Here's how the part is built. I have some questions about the finished solid (model axes, mm). Face numbers are marked on the shaded views. A direction names the side the tool comes from. Coordinates: 2 decimals unless noted, no trailing zeros. Write each loop counter-clockwise with the first axis right and the second up, starting at its lowest first coordinate (ties: lowest second). Pieces come first, ordered by that corner, then holes.
(1) Thinking about a two-plate mould opening in X: for the marked faces 3, 4, 5 and 6, which applies, released by +X, released by -X, zero draft, split by the parting line, or undercut?
(2) For pin 1 Ø3 at (y, z) = (2.5, -25) entering from +X; pin 2 Ø5 at (x, y) = (0, 4.5) entering from +Z; pin 3 Ø1.9 at (x, z) = (-24.5, -20) entering from +Y, each with a flat end and sliding along its axis, tell me the tip position at first contact or that it passes through.
(3) Imagine slicing it at B-B, the plane x = -24.5. List the corners of the cut face in (y, z) for me.
(4) Imagine slicing it at C-C, the plane y = 4.75. List the corners of the cut face in (x, z) for me, plus the area to 3 significant figures.
(5) Imagine slicing it at D-D, the plane x = -45. List the corners of the cut face in (y, z) for me, plus the area to 3 significant figures.
(6) Imagine slicing it at A-A, the plane z = 2.5. List the corners of the cut face in (x, y) for me, plus the area to 3 significant figures.
(7) Please list where these lines run through material, in increasing order: probe 1 along Z at (x, y) = (-7.5, 1); probe 2 along X at (y, z) = (5, 10.5); probe 3 along X at (y, z) = (5.75, -15).
(8) Which directions (+Z, -Z, +X, -X, +Y, -Y) give clear straight access to the entire face, cutting with the end or side of a thin tool? Please do the marked faces 1 and 2.
```python
from build123d import *

# Parameters (mm, degrees)
SKETCH1_R           = 50
BOSS_EXTRUDE1_DEPTH = 10
CUT_EXTRUDE1_DEPTH  = 35
SKETCH5_W           = 35.6075
SKETCH5_H           = 50.6
CUT_EXTRUDE2_DEPTH  = 2.5
SKETCH7_R           = 4.5
CUT_EXTRUDE3_DEPTH  = 10
SKETCH7_3_R         = 4.5
CUT_EXTRUDE4_DEPTH  = 10
SKETCH7_4_R         = 4.5
CUT_EXTRUDE5_DEPTH  = 10


with BuildPart() as part:
    # Sketch1 → Boss-Extrude1 (new body)
    with BuildSketch(Plane(origin=(0, 0, 0), x_dir=(1, 0, 0), z_dir=(0, 1, 0))):
        with Locations(Location((-8.682864084, 10.831764098, 0), (0, 0, 270))):
            Circle(SKETCH1_R)
    extrude(amount=BOSS_EXTRUDE1_DEPTH)

    # Sketch2 → Cut-Extrude1 (cut)
    with BuildSketch(Plane(origin=(0, 10, 0), x_dir=(1, 0, 0), z_dir=(0, 1, 0))):
        with BuildLine():
            Line((-26.490364084, 15.731764356), (-26.492864056, -20.667823814))
            ThreePointArc((-26.492864056, -20.667823814), (-26.308368402, -21.704061868), (-25.777306707, -22.612798037))
            Line((-25.777306707, -22.612798037), (-22.287306707, -26.712798037))
            ThreePointArc((-22.287306707, -26.712798037), (-21.261099672, -27.491624086), (-20.002864084, -27.768235902))
            Line((-20.002864084, -27.768235902), (2.632135916, -27.768235902))
            ThreePointArc((2.632135916, -27.768235902), (3.890371505, -27.491624086), (4.91657854, -26.712798037))
            Line((4.91657854, -26.712798037), (8.40657854, -22.612798037))
            ThreePointArc((8.40657854, -22.612798037), (8.937569086, -21.704255238), (9.122135916, -20.668235902))
            Line((9.122135916, -20.668235902), (9.122135916, 15.721764098))
            ThreePointArc((9.122135916, 15.721764098), (8.938191307, 16.756090949), (8.40891456, 17.663578567))
            Line((8.40891456, 17.663578567), (4.91891456, 21.773578567))
            ThreePointArc((4.91891456, 21.773578567), (3.892008249, 22.554395492), (2.632135916, 22.831764098))
            Line((2.632135916, 22.831764098), (-19.997864084, 22.831764098))
            ThreePointArc((-19.997864084, 22.831764098), (-21.255584517, 22.555390231), (-22.28157091, 21.777190306))
            Line((-22.28157091, 21.777190306), (-25.774070917, 17.677396608))
            ThreePointArc((-25.774070917, 17.677396608), (-26.30563684, 16.768425583), (-26.490364084, 15.731764356))
        make_face()
    extrude(amount=-CUT_EXTRUDE1_DEPTH, mode=Mode.SUBTRACT)

    # Sketch5 → Cut-Extrude2 (cut)
    with BuildSketch(Plane(origin=(0, 10, 0), x_dir=(1, 0, 0), z_dir=(0, 1, 0))):
        with Locations((-8.686614084, -2.468235902)):
            Rectangle(SKETCH5_W, SKETCH5_H)
    extrude(amount=-CUT_EXTRUDE2_DEPTH, mode=Mode.SUBTRACT)

    # Sketch7 → Cut-Extrude3 (cut)
    with BuildSketch(Plane(origin=(0, 10, 0), x_dir=(1, 0, 0), z_dir=(0, 1, 0))):
        with Locations(Location((26.391164769, -9.418235902, 0), (0, 0, 270))):
            Circle(SKETCH7_R)
    extrude(amount=-CUT_EXTRUDE3_DEPTH, mode=Mode.SUBTRACT)

    # Sketch7_3 → Cut-Extrude4 (cut)
    with BuildSketch(Plane(origin=(0, 10, 0), x_dir=(1, 0, 0), z_dir=(0, 1, 0))):
        with Locations(Location((-43.756892937, -9.418235902, 0), (0, 0, 270))):
            Circle(SKETCH7_3_R)
    extrude(amount=-CUT_EXTRUDE4_DEPTH, mode=Mode.SUBTRACT)

    # Sketch7_4 → Cut-Extrude5 (cut)
    with BuildSketch(Plane(origin=(0, 10, 0), x_dir=(1, 0, 0), z_dir=(0, 1, 0))):
        with Locations(Location((-8.682864084, 51.331764098, 0), (0, 0, 270))):
            Circle(SKETCH7_4_R)
    extrude(amount=-CUT_EXTRUDE5_DEPTH, mode=Mode.SUBTRACT)


solid = part.part
```
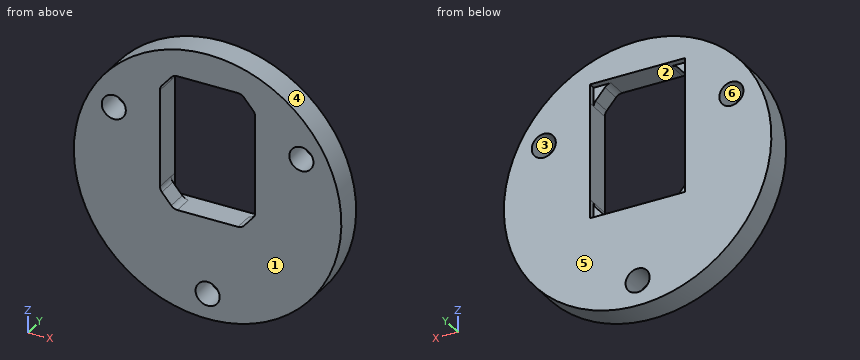
Recorded:
1. face 3: undercut
1. face 4: split by the parting line
1. face 5: zero draft
1. face 6: undercut
2. pin 1: stops at x = 39.69
2. pin 2: stops at z = 38.78
2. pin 3: stops at y = 7.5
3. outline: (0, -58.26) - (10, -58.26) - (10, -22.83) - (7.5, -22.83) - (7.5, -19.17) - (0, -19.17) - close; (0, 24.11) - (7.5, 24.11) - (7.5, 27.77) - (10, 27.77) - (10, 36.6) - (0, 36.6) - close
4. outline: circle Ø100 at (-8.68, -10.83); hole circle Ø9 at (-43.76, 9.42); hole (-26.49, -15.73) arc R3 ccw to (-25.77, -17.68) - (-22.28, -21.78) arc R3 ccw to (-20, -22.83) - (2.63, -22.83) arc R3 ccw to (4.92, -21.77) - (8.41, -17.66) arc R3 ccw to (9.12, -15.72) - (9.12, 20.67) arc R3 ccw to (8.41, 22.61) - (4.92, 26.71) arc R3 ccw to (2.63, 27.77) - (-20, 27.77) arc R3 ccw to (-22.29, 26.71) - (-25.78, 22.61) arc R3 ccw to (-26.49, 20.67) - close; hole circle Ø9 at (-8.68, -51.33); hole circle Ø9 at (26.39, 9.42)
4. area: 5,920 mm2
5. outline: (0, -45.2) - (10, -45.2) - (10, 5.09) - (0, 5.09) - close; (0, 13.74) - (10, 13.74) - (10, 23.53) - (0, 23.53) - close
5. area: 601 mm2
6. outline: (-56.87, 0) - (-26.49, 0) - (-26.49, 10) - (-56.87, 10) - close; (9.12, 0) - (39.51, 0) - (39.51, 10) - (9.12, 10) - close
6. area: 608 mm2
7. probe 1: z = -60.82 to -55.67, -46.99 to -22.83, 27.77 to 39.15
7. probe 2: x = -53.9 to -48.12, -39.39 to -26.49, 9.12 to 22.02, 30.76 to 36.54
7. probe 3: x = -58.51 to -26.49, 9.12 to 41.14
8. face 1: +Z, -Z, +X, -X, -Y
8. face 2: +Y
